Autodesk Inventor part; units mm, degrees
ref_plane "YZ Plane" through (0, 0, 0) normal (1, 0, 0) x (0, 1, 0)
ref_plane "XZ Plane" through (0, 0, 0) normal (0, 1, 0) x (-1, 0, 0)
ref_plane "XY Plane" through (0, 0, 0) normal (0, 0, 1) x (1, 0, 0)
sketch "Sketch1" plane through (0, 0, 0) normal (1, 0, 0) x (0, 1, 0)
  line L0 (21.2, 0) -> (21.2, -3)
  line L1 (42.4, 0) -> (42.4, -3)
  line L2 (63.6, 0) -> (63.6, -3)
  line L3 (84.8, 0) -> (84.8, -3)
  line L4 (-3, -21.2) -> (3, -21.2)
  line L5 (-3, -42.4) -> (3, -42.4)
  line L6 (-3, -63.6) -> (3, -63.6)
  line L7 (-3, -84.8) -> (3, -84.8)
  line L8 (21.2, -106) -> (21.2, -103)
  line L9 (42.4, -106) -> (42.4, -103)
  line L10 (63.6, -106) -> (63.6, -103)
  line L11 (84.8, -106) -> (84.8, -103)
  line L12 (109, -84.8) -> (103, -84.8)
  line L13 (109, -63.6) -> (103, -63.6)
  line L14 (109, -42.4) -> (103, -42.4)
  line L15 (109, -21.2) -> (103, -21.2)
  line L16 (3, -103) -> (3, -84.8)
  line L17 (3, -63.6) -> (3, -42.4)
  line L18 (3, -21.2) -> (3, -3)
  line L19 (103, -3) -> (103, -21.2)
  line L20 (103, -42.4) -> (103, -63.6)
  line L21 (103, -84.8) -> (103, -103)
  line L22 (21.2, -103) -> (3, -103)
  line L23 (84.8, -106) -> (63.6, -106)
  line L24 (42.4, -106) -> (21.2, -106)
  line L25 (103, -103) -> (84.8, -103)
  line L26 (63.6, -103) -> (42.4, -103)
  line L27 (103, -3) -> (103, 0)
  line L28 (3, -3) -> (3, 0)
  line L29 (3, 0) -> (21.2, 0)
  line L30 (21.2, -3) -> (42.4, -3)
  line L31 (63.6, -3) -> (84.8, -3)
  line L32 (42.4, 0) -> (63.6, 0)
  line L33 (84.8, 0) -> (103, 0)
  line L34 (-3, -63.6) -> (-3, -84.8)
  line L35 (-3, -21.2) -> (-3, -42.4)
  line L36 (109, -21.2) -> (109, -42.4)
  line L37 (109, -63.6) -> (109, -84.8)
  line L38 (-1, -26.8) -> (0, -26.8)
  line L39 (0, -26.8) -> (0, -36.8)
  line L40 (0, -36.8) -> (-1, -36.8)
  line L41 (-1, -36.8) -> (-1, -26.8)
  line L42 (0, -79.2) -> (-1, -79.2)
  line L43 (-1, -79.2) -> (-1, -69.2)
  line L44 (-1, -69.2) -> (0, -69.2)
  line L45 (0, -69.2) -> (0, -79.2)
  line L46 (106, -26.8) -> (107, -26.8)
  line L47 (107, -26.8) -> (107, -36.8)
  line L48 (107, -36.8) -> (106, -36.8)
  line L49 (106, -36.8) -> (106, -26.8)
  line L50 (106, -69.2) -> (105, -69.2)
  line L51 (105, -69.2) -> (105, -79.2)
  line L52 (105, -79.2) -> (106, -79.2)
  line L53 (106, -79.2) -> (106, -69.2)
  point P0 (0, 0)
  dimension "d109" = 10
  dimension "d110" = 10
  dimension "d111" = 1
  dimension "d112" = 10
  dimension "d113" = 1
  dimension "d114" = 10
extrude "Extrusion1" add sketch "Sketch1" along normal blind 3
sketch "Sketch3" plane through (3, 0, 0) normal (1, 0, 0) x (0, 0, -1)
  circle A0 centre (53, 53) radius 5
  point P0 (0, 0)
  dimension "d6" = 10
hole "Hole1" at (3, 53, -53) direction (-1, 0, 0) diameter 15 end through all
sketch "Sketch5" plane through (3, 0, 0) normal (1, 0, 0) x (0, 0, -1)
  circle A0 centre (25, 20) radius 1.5
  point P0 (0, 0)
  dimension "d45" = 3
hole "Hole4" at (3, 20, -25) direction (-1, 0, 0) diameter 3 end through all
sketch "Sketch6" plane through (3, 0, 0) normal (1, 0, 0) x (0, 0, -1)
  circle A0 centre (53, 20) radius 1.5
  point P0 (0, 0)
  dimension "d53" = 3
sketch "Sketch7" plane through (3, 0, 0) normal (1, 0, 0) x (0, 0, -1)
  point P0 (0, 0)
hole "Hole5" at (3, 20, -53) direction (-1, 0, 0) diameter 3 end through all
sketch "Sketch8" plane through (3, 0, 0) normal (1, 0, 0) x (0, 0, -1)
  circle A0 centre (81, 20) radius 1.5
  point P0 (0, 0)
  dimension "d61" = 3
hole "Hole6" at (3, 20, -81) direction (-1, 0, 0) diameter 3 end through all
sketch "Sketch9" plane through (3, 0, 0) normal (1, 0, 0) x (0, 0, -1)
  circle A0 centre (25, 53) radius 1.5
  point P0 (0, 0)
  dimension "d69" = 3
hole "Hole7" at (3, 53, -25) direction (-1, 0, 0) diameter 3 end through all
sketch "Sketch10" plane through (3, 0, 0) normal (1, 0, 0) x (0, 0, -1)
  circle A0 centre (81, 53) radius 1.5
  point P0 (0, 0)
  dimension "d77" = 3
hole "Hole8" at (3, 53, -81) direction (-1, 0, 0) diameter 3 end through all
sketch "Sketch11" plane through (3, 0, 0) normal (1, 0, 0) x (0, 0, -1)
  circle A0 centre (25, 86) radius 1.5
  point P0 (0, 0)
  dimension "d85" = 3
hole "Hole9" at (3, 86, -25) direction (-1, 0, 0) diameter 3 end through all
sketch "Sketch12" plane through (3, 0, 0) normal (1, 0, 0) x (0, 0, -1)
  circle A0 centre (53, 86) radius 1.5
  point P0 (0, 0)
  dimension "d93" = 3
hole "Hole10" at (3, 86, -53) direction (-1, 0, 0) diameter 3 end through all
sketch "Sketch13" plane through (3, 0, 0) normal (1, 0, 0) x (0, 0, -1)
  circle A0 centre (81, 86) radius 1.5
  point P0 (0, 0)
  dimension "d101" = 3
hole "Hole11" at (3, 86, -81) direction (-1, 0, 0) diameter 3 end through all
properties part number "Box side 1" material "PMMA Plastic"
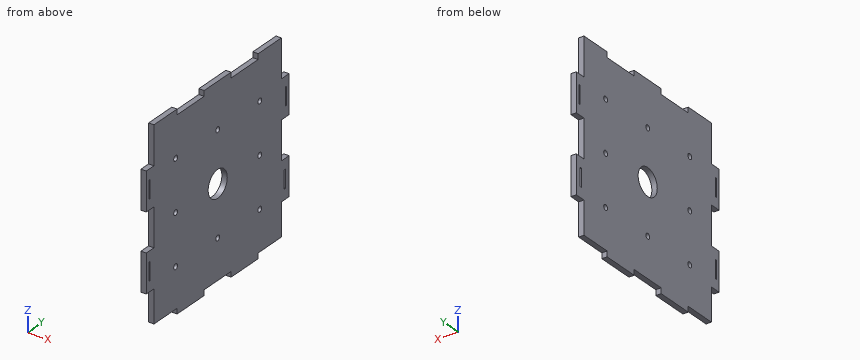
Source: CAD feature listing. Evaluate the final solid. Frame: model axes, mm. Give positions to 0.01 mm unless a question says otherwise; leave off trailing zeros. Write each loop counter-clockwise with the first axis right and the second up, starting at its lowest first coordinate (ties: lowest second). Pieces come first, ordered by that corner, then holes.
1. Material intervals for line 1 along Y through (x, z) = (1.35, -81); line 2 along Z through (x, y) = (1.65, 86); line 3 along Y through (x, z) = (1.95, -75), sorted ascending.
2. Section query C-C (z = -81). Return the cut outline in (x, y), then the cut area to 3 significant figures.
3. Section query A-A (z = -53). Return the cut outline in (x, y), then the cut area to 3 significant figures.
4. First-contact query: pin 1 (1.5 mm diameter, centred on x = 1.5, y = 15.5, fed in from -Z); pin 2 (1.1 mm diameter, centred on x = 2, y = -0.5, fed in from -Z); pin 3 (0.8 mm diameter, centred on x = 1.5, y = 106.5, fed in from +Z). Flat tips, straight axial feed; report the tip coordinate or a pass-through.
5. Section query B-B (y = 101). Return the cut outline in (x, z), then the cut area to 3 significant figures.
Output values:
1. line 1: y = -3 to 18.5, 21.5 to 51.5, 54.5 to 84.5, 87.5 to 109
1. line 2: z = -103 to -82.5, -79.5 to -54.5, -51.5 to -26.5, -23.5 to 0
1. line 3: y = -3 to -1, 0 to 105, 106 to 109
2. outline: (0, -3) - (3, -3) - (3, 18.5) - (0, 18.5) - close; (0, 21.5) - (3, 21.5) - (3, 51.5) - (0, 51.5) - close; (0, 54.5) - (3, 54.5) - (3, 84.5) - (0, 84.5) - close; (0, 87.5) - (3, 87.5) - (3, 109) - (0, 109) - close
2. area: 309 mm2
3. outline: (0, 3) - (3, 3) - (3, 18.5) - (0, 18.5) - close; (0, 21.5) - (3, 21.5) - (3, 45.5) - (0, 45.5) - close; (0, 60.5) - (3, 60.5) - (3, 84.5) - (0, 84.5) - close; (0, 87.5) - (3, 87.5) - (3, 103) - (0, 103) - close
3. area: 237 mm2
4. pin 1: stops at z = -103
4. pin 2: stops at z = -84.8
4. pin 3: stops at z = -21.2
5. outline: (0, -103) - (3, -103) - (3, 0) - (0, 0) - close
5. area: 309 mm2
